Autodesk Inventor part; units mm, degrees
ref_plane "YZ Plane" through (0, 0, 0) normal (1, 0, 0) x (0, 1, 0)
ref_plane "XZ Plane" through (0, 0, 0) normal (0, 1, 0) x (-1, 0, 0)
ref_plane "XY Plane" through (0, 0, 0) normal (0, 0, 1) x (1, 0, 0)
sketch "Sketch1" plane through (0, 0, 0) normal (0, 0, 1) x (1, 0, 0)
  circle A0 centre (0, 0) radius 10
  circle A1 centre (0, 0) radius 30
  circle A2 centre (340, 0) radius 10
  circle A3 centre (340, 0) radius 30
  line L0 (0, 38) -> (340, 38)
  arc A4 (340, -38) -> (340, 38) centre (340, 0) ccw
  line L1 (340, -38) -> (0, -38)
  arc A5 (0, 38) -> (0, -38) centre (0, 0) ccw
  line L2 (340, 30) -> (0, 30)
  arc A6 (0, 30) -> (0, -30) centre (0, 0) ccw
  line L3 (0, -30) -> (340, -30)
  arc A7 (340, -30) -> (340, 30) centre (340, 0) ccw
  dimension "d0" = 8
extrude "Extrusion1" add sketch "Sketch1" against normal blind 8 contours L0 A4 L1 A5
properties part number "ketting1"
The model under review builds one solid part; all positions refer to its coordinate system, in mm. A direction names the side the tool comes from. Coordinates: 2 decimals unless noted, no trailing zeros. Loops run counter-clockwise (first coordinate to the right, second up) from the corner with the lowest first, then second, coordinate; pieces in that order, holes last. Notation, with made-up numbers: (-22.5, 67.5) -> (11.5, 67.5) arc R9 cw to (11.5, 79.5) -> close; hole circle Ø10 at (69.25, -16). An arc over 180 degrees is marked (long way). Use a Markdown table: item, result. Add a question column.
1. Machinability: for faces 4 (the face through (168, 38, -4)), 5 (the face through (-29.993, 0.66, -3.944)), which of the approach directions +Z, -Z, +X, -X, +Y, -Y give a long, thin tool a straight path to every point of the face, cutting with its end or side? Answer none if there is none.
2. Add section C-C on z = -5. Write out the cut boundary in (x, y).
3. Add section B-B on y = 0. Write out the cut boundary in (x, z).
4. Add section A-A on x = 112. Write out the cut boundary in (y, z).
5. To check wall thickness, follow line 1 (Y direction, x = 117, z = -3.5); line 2 (X direction, y = 1, z = -4); line 3 (X direction, y = -8.5, z = -4.25). State the ranges of each line that lie inside material, in increasing order.
6. Draft analysis for pull direction Y (two halves, no side actions). For faces 1 (the face through (169, 31, -8)), 2 (the face through (377.99, -0.84, -3.94)), 3 (the face through (172, 30, -4)), state which applies: pulls with the +Y half, pulls with the -Y half, needs draft (parallel to the pull), parting line crosses it, or undercut.
7. Clearance check with flat-ended pins moving along their axes: pin 1 Ø1 at (y, z) = (5, -3) entering from -X; pin 2 Ø1 at (y, z) = (1.5, -7) entering from -X; pin 3 Ø1 at (y, z) = (19, -3.5) entering from -X. State where each tip first meets the part, or that it passes through.
Returned:
| question | item | result |
|---|---|---|
| 1 | face 4 | +Z, -Z, +X, -X, +Y |
| 1 | face 5 | +Z, -Z |
| 2 | outline | (0, -38) -> (340, -38) arc R38 ccw to (340, 38) -> (0, 38) arc R38 ccw to start; hole (0, -30) -> (340, -30) arc R30 ccw to (340, 30) -> (0, 30) arc R30 ccw to start |
| 3 | outline | (-38, -8) -> (-30, -8) -> (-30, 0) -> (-38, 0) -> close; (370, -8) -> (378, -8) -> (378, 0) -> (370, 0) -> close |
| 4 | outline | (-38, -8) -> (-30, -8) -> (-30, 0) -> (-38, 0) -> close; (30, -8) -> (38, -8) -> (38, 0) -> (30, 0) -> close |
| 5 | line 1 | y = -38 to -30, 30 to 38 |
| 5 | line 2 | x = -37.99 to -29.98, 369.98 to 377.99 |
| 5 | line 3 | x = -37.04 to -28.77, 368.77 to 377.04 |
| 6 | face 1 | needs draft |
| 6 | face 2 | parting line crosses it |
| 6 | face 3 | undercut |
| 7 | pin 1 | stops at x = -37.73 |
| 7 | pin 2 | stops at x = -37.99 |
| 7 | pin 3 | stops at x = -33.19 |
